Source: CAD feature listing. Evaluate the final solid. Frame: model axes, mm. Face numbers are marked on the shaded views. A direction names the side the tool comes from. Round coordinates to 2 decimals unless told otherwise and drop trailing zeros. Put each result on its own line as item: value. Start each with the question number.
1) Line query: probe 1 along Y at (x, z) = (0, 8.25); probe 2 along X at (y, z) = (-12, 8); probe 3 along Y at (x, z) = (-5.5, 5.75). Output: solid intervals per line, ascending. Write a range as [from, to].
2) Contact query for flat-ended pins moving along their axis: P1, Ø5, axis at y = 12, z = 2.5, coming from the +X side; P2, Ø2, axis at y = -11, z = 7, coming from the +X side; P3, Ø1, axis at y = 10, z = 15, coming from the +X side. Output: stop coordinate, or through.
3) Mould query, pull axis Z, two halves, no side actions, for the marked faces 6, 7 and 8. Classes: +Z half, -Z half, draft (parallel to the pull), parting line (faces both ways), or undercut.
4) Access query for the marked faces 1, 2, 3, 4 and 5. Directions: +Z, -Z, +X, -X, +Y, -Y. A direction counts if a zero-diameter tool reaches every point of the face in a straight line with its end or side. Return the directions, or none.
```python
from build123d import *

# Parameters (mm, degrees)
BOSS_EXTRUDE1_DEPTH = 20
SKETCH5_OUTSIDE_W   = 154.97
SKETCH5_OUTSIDE_H   = 154.97
SKETCH5_OUTSIDE_R   = 22.5
CUT_EXTRUDE1_DEPTH  = 20
CUT_EXTRUDE1_TAPER  = 60
SKETCH6_R           = 15
CUT_EXTRUDE2_DEPTH  = 21


with BuildPart() as part:
    # Sketch1 → Boss-Extrude1 (new body)
    with BuildSketch(Plane.XY):
        Polygon((22.5, -12.990381057), (22.5, 12.990381057), (0, 25.980762114), (-22.5, 12.990381057), (-22.5, -12.990381057), (0, -25.980762114), align=None)
    extrude(amount=BOSS_EXTRUDE1_DEPTH)

    # Sketch2 → Revolve1 (revolve)
    with BuildSketch(Plane(origin=(0, 0, 0), x_dir=(0, 0, -1), z_dir=(1, 0, 0))):
        with BuildLine():
            Line((0, 0), (-12, 0))
            ThreePointArc((-12, 0), (-10.89665903, -17.717879555), (-0.820783292, -32.333533674))
            ThreePointArc((-0.820783292, -32.333533674), (-0.288330028, -32.402985456), (0, -31.95))
            Line((0, -31.95), (0, 0))
        make_face()
    revolve(axis=Axis((0, 0, 0), (0, 0, 1)))

    # Sketch5 outside → Cut-Extrude1 (cut)
    with BuildSketch(Plane.XY.offset(20)):
        Rectangle(SKETCH5_OUTSIDE_W, SKETCH5_OUTSIDE_H)
        Circle(SKETCH5_OUTSIDE_R, mode=Mode.SUBTRACT)
    extrude(amount=-CUT_EXTRUDE1_DEPTH, taper=CUT_EXTRUDE1_TAPER, mode=Mode.SUBTRACT)

    # Sketch6 → Cut-Extrude2 (cut, through all)
    with BuildSketch(Plane.XY.offset(20)):
        Circle(SKETCH6_R)
    extrude(amount=-CUT_EXTRUDE2_DEPTH, mode=Mode.SUBTRACT)


solid = part.part
```
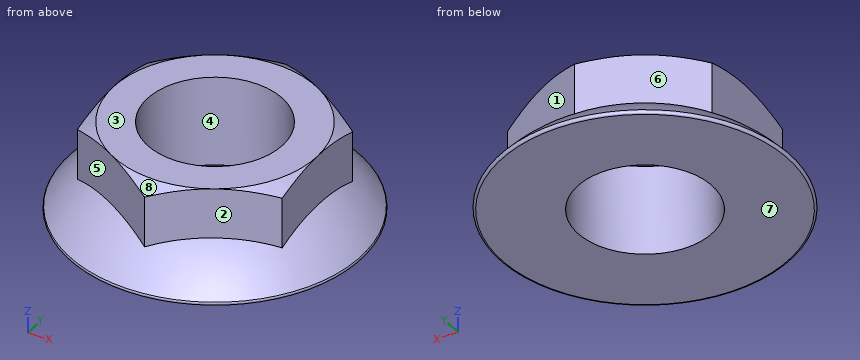
Answer sheet:
1. probe 1: [-25.98, -15], [15, 25.98]
1. probe 2: [-22.5, -9], [9, 22.5]
1. probe 3: [-26.66, -13.96], [13.96, 26.66]
2. P1: x = 30.74
2. P2: x = 24.61
2. P3: x = 22.5
3. face 6: draft
3. face 7: -Z half
3. face 8: +Z half
4. face 1: +Z, +X, +Y
4. face 2: +Z, +X, -Y
4. face 3: +Z, +X, -X, +Y, -Y
4. face 4: +Z, -Z
4. face 5: +Z, -X, -Y
